The drawing under review shows one solid part. Ordinate dimensions are in mm from its lowest x, y, z. A direction names the side the tool comes from. Coordinates: 2 decimals unless noted, no trailing zeros. Order: outer loops, then holes, each group sorted by start corner. A loop starts at its lowest first (then second) coordinate and runs counter-clockwise, first axis right, second up.
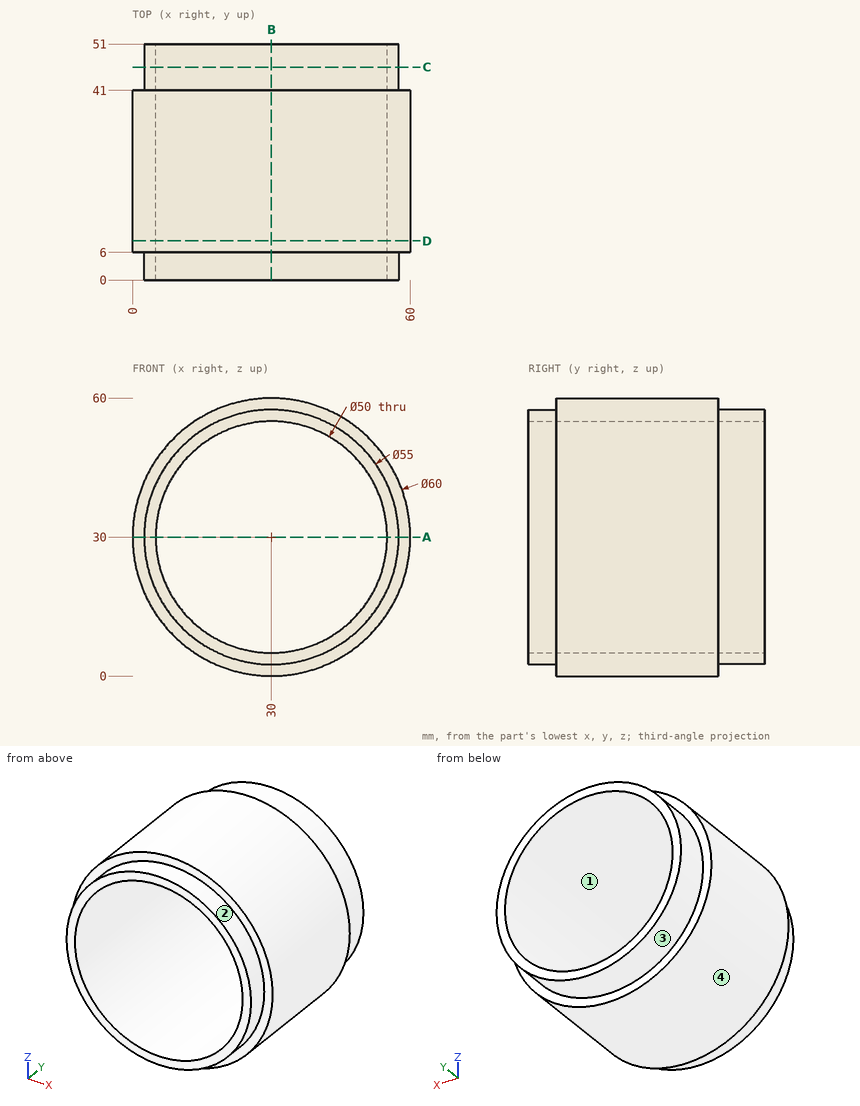
(1) We need section A-A, the plane z = 30. Write out the cut boundary in (x, y).
A:
outline: (0, 6) - (2.5, 6) - (2.5, 0) - (5, 0) - (5, 51) - (2.5, 51) - (2.5, 41) - (0, 41) - close; (55, 0) - (57.5, 0) - (57.5, 6) - (60, 6) - (60, 41) - (57.5, 41) - (57.5, 51) - (55, 51) - close
(2) We need section B-B, the plane x = 30. Write out the cut boundary in (y, z), and give its area (3 significant figures).
A:
outline: (0, 2.5) - (6, 2.5) - (6, 0) - (41, 0) - (41, 2.5) - (51, 2.5) - (51, 5) - (0, 5) - close; (0, 55) - (51, 55) - (51, 57.5) - (41, 57.5) - (41, 60) - (6, 60) - (6, 57.5) - (0, 57.5) - close
area: 430 mm2
(3) We need section D-D, the plane y = 8.5. Write out the cut boundary in (x, z).
A:
outline: circle Ø60 at (30, 30); hole circle Ø50 at (30, 30)
(4) For pin 1 Ø1.5 at (x, y) = (33, 43.5) entering from +Z; pin 2 Ø4 at (x, y) = (37.5, 5) entering from -Z; pin 3 Ø8 at (y, z) = (8.5, 8) entering from +X, all flat-tipped, find the tip position at first contact; note any pin that passes through.
A:
pin 1: stops at z = 57.41
pin 2: stops at z = 0.56
pin 3: stops at x = 54
(5) Draft analysis for pull direction X (two halves, no side actions). For the marked faces 1 and 2, state which applies: released by +X, released by -X, zero draft, split by the parting line, or undercut.
A:
face 1: undercut
face 2: split by the parting line
(6) We need section C-C, the plane y = 46. Write out the cut boundary in (x, z), and give its area (3 significant figures).
A:
outline: circle Ø55 at (30, 30); hole circle Ø50 at (30, 30)
area: 412 mm2
(7) Wall thickness on probe 1 along Z at (x, y) = (30, 17); probe 2 along X at (y, z) = (16, 48.5); probe 3 along X at (y, z) = (12.5, 43): over which ranges is each line inside the solid? List them lowest first.
A:
probe 1: z = 0 to 5, 55 to 60
probe 2: x = 6.38 to 13.18, 46.82 to 53.62
probe 3: x = 2.96 to 8.65, 51.35 to 57.04
(8) Machinability: for the marked faces 3 and 4, which of the approach directions +Z, -Z, +X, -X, +Y, -Y give a long, thin tool a straight path to every point of the face, cutting with its end or side? Answer none if there is none.
A:
face 3: +Y
face 4: +Y, -Y
